Study the drawing (mm; zero at the part's minimum x, y, z) and answer. Give positions to 0.01 mm unless a question says otherwise; leave off trailing zeros. Order: outer loops, then holes, each group sorted by start corner. A loop starts at its lowest first (then second) coordinate and runs counter-clockwise, first axis right, second up. Notation, with made-up numbers: (-8.5, -18) - (18.5, -18) arc R37 cw to (18.5, 20) - close; hole circle Ø9 at (21, 4). An arc over 180 degrees is marked (long way). Return JSON: item names as keys, results as strings.
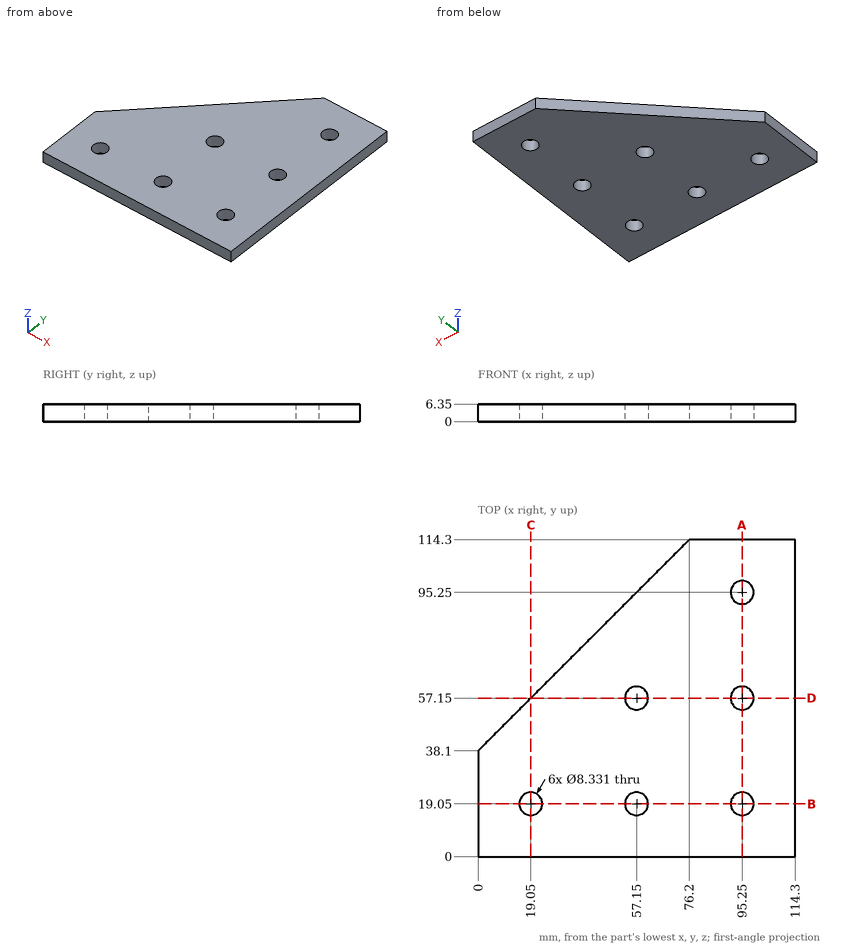
Q1. A cutting plane is placed at C-C (x = 19.05). Write down the section's boundary in (y, z).
Values:
{"outline": "(0, 0) - (14.88, 0) - (14.88, 6.35) - (0, 6.35) - close; (23.22, 0) - (57.15, 0) - (57.15, 6.35) - (23.22, 6.35) - close"}
Q2. A cutting plane is placed at D-D (y = 57.15). Write down the section's boundary in (x, z), and give its area (3 significant figures).
Values:
{"outline": "(19.05, 0) - (52.98, 0) - (52.98, 6.35) - (19.05, 6.35) - close; (61.32, 0) - (91.08, 0) - (91.08, 6.35) - (61.32, 6.35) - close; (99.42, 0) - (114.3, 0) - (114.3, 6.35) - (99.42, 6.35) - close", "area": "499 mm²"}
Q3. Given pin 1 (1 mm diameter, centred on x = 48, z = 3.5, fed in from +Y); pin 2 (7.5 mm diameter, centred on x = 57.15, y = 57.15, fed in from +Z) (1 decimal); pin 3 (1 mm diameter, centred on x = 30.5, z = 4, fed in from +Y); pin 4 (1 mm diameter, centred on y = 97.5, z = 3.5, fed in from -X), each flat-ended and moving along its own axis, determine where each tip first touches the part or whether it passes through.
Values:
{"pin 1": "stops at y = 86.6", "pin 2": "passes through", "pin 3": "stops at y = 69.1", "pin 4": "stops at x = 58.9"}
Q4. Consider L1, parallel to Y at x = 95, z = 5; L2, parallel to Y at x = 91.5, z = 2.75 (1 decimal); L3, parallel to Y at x = 56, z = 2. Determine where each line is inside the solid, lowest interval first.
Values:
{"L1": "y = 0 to 14.89, 23.21 to 52.99, 61.31 to 91.09, 99.41 to 114.3", "L2": "y = 0 to 17.2, 20.9 to 55.3, 59 to 93.4, 97.1 to 114.3", "L3": "y = 0 to 15.05, 23.05 to 53.15, 61.15 to 94.1"}
Q5. A cutting plane is placed at A-A (x = 95.25). Write down the section's boundary in (y, z).
Values:
{"outline": "(0, 0) - (14.88, 0) - (14.88, 6.35) - (0, 6.35) - close; (23.22, 0) - (52.98, 0) - (52.98, 6.35) - (23.22, 6.35) - close; (61.32, 0) - (91.08, 0) - (91.08, 6.35) - (61.32, 6.35) - close; (99.42, 0) - (114.3, 0) - (114.3, 6.35) - (99.42, 6.35) - close"}
